Answer from the drawing. Dimensions are ordinates in mm from the lowest x, y and z of the part. Round coordinates to 2 decimals unless told otherwise and drop trailing zeros. Loops run counter-clockwise (first coordinate to the right, second up) from the corner with the lowest first, then second, coordinate; pieces in that order, holes last. Notation, with made-up numbers: (55, 50.25) - (77, 50.25) arc R31 cw to (77, 87.25) - close; hole circle Ø2 at (43, 86.25). An arc over 180 degrees is marked (long way). Return JSON: item names as keys, results as strings.
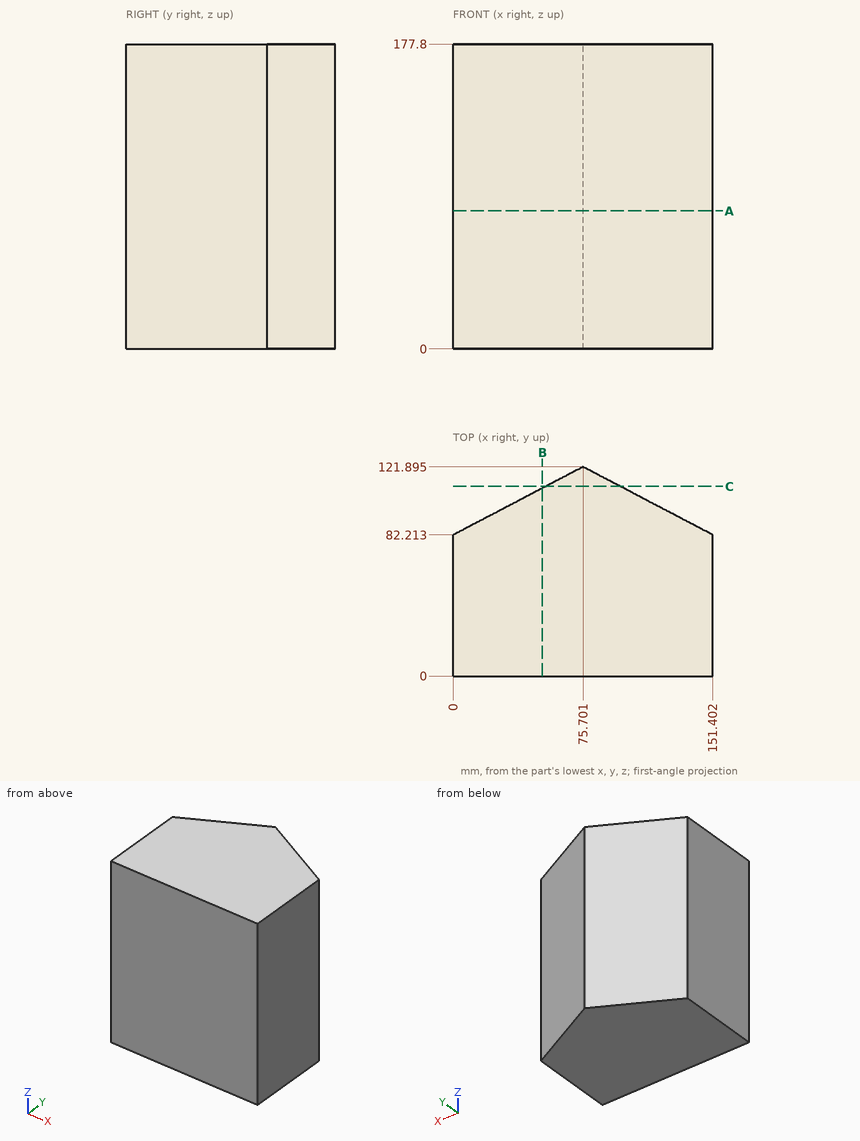
1) Section C-C (y = 110.5) is taken. Give the vertices of the cut face in (x, z), and give its area (3 significant figures).
Verdict:
{"outline": "(53.96, 0) - (97.44, 0) - (97.44, 177.8) - (53.96, 177.8) - close", "area": "7,730 mm2"}
2) Section A-A (z = 80.5) is taken. Give the vertices of the cut face in (x, y) (1 decimal).
Verdict:
{"outline": "(0, 0) - (151.4, 0) - (151.4, 82.2) - (75.7, 121.9) - (0, 82.2) - close"}
3) Flat-ended cylindrical pins translate along their axes: pin 1 (4 mm diameter, centred on x = 36, z = 70.5, fed in from +Y); pin 2 (1 mm diameter, centred on y = 107.5, z = 105.5, fed in from -X) (1 decimal). Find the tip coordinate at first contact, or state that the pin passes through.
Verdict:
{"pin 1": "stops at y = 102.13", "pin 2": "stops at x = 47.3"}
4) Find the intervals of material crossed by L1, parallel to Y at x = 22.5, z = 44.5; L2, parallel to Y at x = 130, z = 93; L3, parallel to X at y = 106, z = 114.5 (1 decimal), in increasing order.
Verdict:
{"L1": "y = 0 to 94.01", "L2": "y = 0 to 93.43", "L3": "x = 45.4 to 106"}
5) Section B-B (x = 52) is taken. Give the vertices of the cut face in (y, z).
Verdict:
{"outline": "(0, 0) - (109.47, 0) - (109.47, 177.8) - (0, 177.8) - close"}
